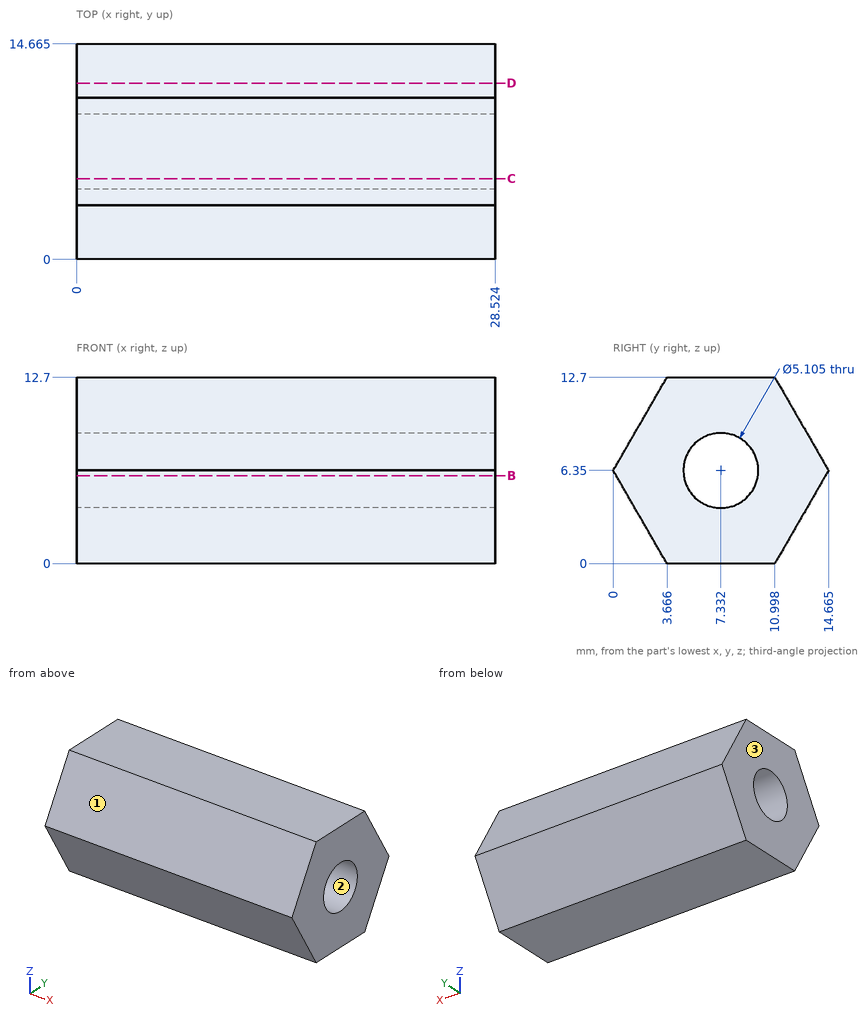
The drawing under review shows one solid part. Ordinate dimensions are in mm from its lowest x, y, z. Round coordinates to 2 decimals unless told otherwise and drop trailing zeros. Loops run counter-clockwise (first coordinate to the right, second up) from the corner with the lowest first, then second, coordinate; pieces in that order, holes last. Notation, with made-up numbers: (31, -2.5) - (44, -2.5) arc R19 cw to (44, 17.5) - close; hole circle Ø1 at (66, -24.75). An arc over 180 degrees is marked (long way). One line per question, with ' | ' between items.
Q1. For line 1 along Y through (x, z) = (1.5, 6.75) (1 decimal); line 2 along Z through (x, y) = (19.5, 5.25) (1 decimal); line 3 along Z through (x, y) = (5.5, 9) (1 decimal), list the stretches that pass through material, from the lowest coordinate up. Write a range as [from, to].
Taken from the geometry:
line 1: y = [0.2, 4.8], [9.9, 14.4] | line 2: z = [0, 4.9], [7.8, 12.7] | line 3: z = [0, 4.4], [8.3, 12.7]
Q2. For pin 1 (4 mm diameter, centred on x = 10.5, z = 2.5, fed in from +Y); pin 2 (1 mm diameter, centred on x = 4.5, z = 7, fed in from +Y); pin 3 (2 mm diameter, centred on x = 21.5, y = 2.5, fed in from -Z) (1 decimal); pin 4 (6 mm diameter, centred on x = 3.5, z = 5, fed in from -Y), all flat-tipped, find the tip position at first contact; note any pin that passes through.
Taken from the geometry:
pin 1: stops at y = 13.6 | pin 2: stops at y = 14.58 | pin 3: stops at z = 0.3 | pin 4: stops at y = 0
Q3. Take a section at C-C (y = 5.5). Give the boundary of the cut face in (x, z) (1 decimal), and give its area (3 significant figures).
Taken from the geometry:
outline: (0, 0) - (28.5, 0) - (28.5, 4.6) - (0, 4.6) - close; (0, 8.1) - (28.5, 8.1) - (28.5, 12.7) - (0, 12.7) - close | area: 261 mm²
Q4. Take a section at D-D (y = 12). Give the boundary of the cut face in (x, z) (1 decimal), and give its area (3 significant figures).
Taken from the geometry:
outline: (0, 1.7) - (28.5, 1.7) - (28.5, 11) - (0, 11) - close | area: 263 mm²
Q5. The part is to be moulded in two halves that separate along Y. For the marked faces 1, 2 and 3, say which applies: released by +Y, released by -Y, zero draft, split by the parting line, or undercut.
Taken from the geometry:
face 1: released by -Y | face 2: undercut | face 3: zero draft
Q6. Take a section at B-B (z = 6). Give the boundary of the cut face in (x, y) (1 decimal).
Taken from the geometry:
outline: (0, 0.2) - (28.5, 0.2) - (28.5, 4.8) - (0, 4.8) - close; (0, 9.9) - (28.5, 9.9) - (28.5, 14.5) - (0, 14.5) - close
